Source: CAD feature listing. Evaluate the final solid. Frame: model axes, mm. Coordinates: 2 decimals unless noted, no trailing zeros. Loops run counter-clockwise (first coordinate to the right, second up) from the corner with the lowest first, then second, coordinate; pieces in that order, holes last. Notation, with made-up numbers: (1, -34.75) -> (31, -34.75) arc R20 cw to (31, -27.75) -> close; hole circle Ø9 at (54, 86). An arc over 180 degrees is marked (long way). Answer as CSV lines item,"result".
from build123d import *

# Parameters (mm, degrees)
SKETCH_1_W      = 124
SKETCH_1_H      = 8
SKETCH_1_R      = 1.5
EXTRUDE_1_DEPTH = 8


with BuildPart() as part:
    # 草图1 → 凸台-拉伸1 (new body)
    with BuildSketch(Plane.XY):
        with Locations((62, 4)):
            Rectangle(SKETCH_1_W, SKETCH_1_H)
        with Locations((62, 4)):
            Circle(SKETCH_1_R, mode=Mode.SUBTRACT)
        with Locations((10, 4)):
            Circle(SKETCH_1_R, mode=Mode.SUBTRACT)
        with Locations(Location((114, 4, 0), (0, 0, 180))):
            Circle(SKETCH_1_R, mode=Mode.SUBTRACT)
    extrude(amount=EXTRUDE_1_DEPTH)


solid = part.part
(1) Cut plane C-C (z = 3.5). Return the cut outline in (x, y), then the cut area to 3 significant figures.
Computed values:
outline,"(0, 0) -> (124, 0) -> (124, 8) -> (0, 8) -> close; hole circle Ø3 at (10, 4); hole circle Ø3 at (62, 4); hole circle Ø3 at (114, 4)"
area,"971 mm^2"
(2) Cut plane B-B (x = 62). Return the cut outline in (y, z).
Computed values:
outline,"(0, 0) -> (2.5, 0) -> (2.5, 8) -> (0, 8) -> close; (5.5, 0) -> (8, 0) -> (8, 8) -> (5.5, 8) -> close"
(3) Draft query along X for faces 1 (the flat face through (61, 8, 4)), 2 (the flat face through (0, 4, 4)), 3 (the cylindrical face through (115.5, 3.93, 3.94)). Return one class per face: released by +X, released by -X, zero draft, split by the parting line, or undercut.
Computed values:
face 1,"zero draft"
face 2,"released by -X"
face 3,"undercut"
(4) Material intervals for L1, parallel to Y at x = 62, z = 2.5; L2, parallel to X at y = 4.75, z = 2.75, sorted ascending. Write a range as [from, to].
Computed values:
L1,"[0, 2.5], [5.5, 8]"
L2,"[0, 8.7], [11.3, 60.7], [63.3, 112.7], [115.3, 124]"
(5) Cut plane A-A (y = 4). Return the cut outline in (x, z).
Computed values:
outline,"(0, 0) -> (8.5, 0) -> (8.5, 8) -> (0, 8) -> close; (11.5, 0) -> (60.5, 0) -> (60.5, 8) -> (11.5, 8) -> close; (63.5, 0) -> (112.5, 0) -> (112.5, 8) -> (63.5, 8) -> close; (115.5, 0) -> (124, 0) -> (124, 8) -> (115.5, 8) -> close"
